Read the model definition and answer for the solid it produces. Units are mm, in the model's axes. A direction names the side the tool comes from. Give positions to 0.01 mm unless a question says otherwise; leave off trailing zeros. Order: outer loops, then holes, each group sorted by start corner. A loop starts at its lowest first (then second) coordinate and runs counter-clockwise, first axis right, second up. Notation, with made-up numbers: M 85,63.25 L 123,63.25 A21 cw 123,93.25 Z; hole C 54,-14.5 d1. An arc over 180 degrees is marked long. One line per item, written item: value.
from build123d import *

# Parameters (mm, degrees)
BOSS_EXTRUDE2_DEPTH = 6


with BuildPart() as part:
    # Sketch1 → Boss-Extrude2 (new body)
    with BuildSketch(Plane(origin=(0, 0, 0), x_dir=(1, 0, 0), z_dir=(0, 1, 0))):
        with BuildLine():
            Line((7.988162854, 331.501326389), (7.988162854, 171.337454215))
            ThreePointArc((7.988162854, 171.337454215), (9.818693497, 167.235107296), (13.984274361, 165.553432905))
            Line((13.984274361, 165.553432905), (49.307855037, 165.553432905))
            Line((49.307855037, 165.553432905), (49.307855037, 163.543518894))
            Line((49.307855037, 163.543518894), (13.984274361, 163.543518894))
            ThreePointArc((13.984274361, 163.543518894), (8.320398521, 165.889579716), (5.974360349, 171.553464938))
            Line((5.974360349, 171.553464938), (5.974999998, 331.501302447))
            ThreePointArc((5.974999998, 331.501302447), (-0.011825567, 337.488163533), (-5.998674291, 331.501325605))
            Line((-5.998674291, 331.501325605), (-5.998674291, 0.561440532))
            ThreePointArc((-5.998674291, 0.561440532), (-0.306028697, -5.993414959), (5.975, 0))
            Line((5.975, 0), (5.975, 115.356719051))
            ThreePointArc((5.975, 115.356719051), (8.250227281, 120.944829403), (13.781744328, 123.354384475))
            Line((13.781744328, 123.354384475), (308.33721248, 123.354384475))
            ThreePointArc((308.33721248, 123.354384475), (313.994066729, 121.011238725), (316.33721248, 115.354384475))
            Line((316.33721248, 115.354384475), (316.33721248, 0.000205216))
            ThreePointArc((316.33721248, 0.000205216), (322.337222061, -5.999794784), (328.33721248, 0.000224379))
            Line((328.33721248, 0.000224379), (328.336683355, 331.50001256))
            ThreePointArc((328.336683355, 331.50001256), (322.26179375, 337.500094056), (316.337490676, 331.351281588))
            Line((316.337490676, 331.351281588), (316.337490676, 171.552255024))
            ThreePointArc((316.337490676, 171.552255024), (313.994332551, 165.895370899), (308.337448427, 163.552212774))
            Line((308.337448427, 163.552212774), (90.793200611, 163.552212774))
            ThreePointArc((90.793200611, 163.552212774), (90.43964722, 163.405766165), (90.293200611, 163.052212774))
            Line((90.293200611, 163.052212774), (90.293200611, 157.424591987))
            Line((90.293200611, 157.424591987), (90.293200611, 154.657877928))
            Line((90.293200611, 154.657877928), (88.293002078, 154.657877928))
            Line((88.293002078, 154.657877928), (88.293002078, 157.424591987))
            Line((88.293002078, 157.424591987), (88.293002078, 163.552212774))
            ThreePointArc((88.293002078, 163.552212774), (88.878788516, 164.966468586), (90.293002078, 165.552255024))
            Line((90.293002078, 165.552255024), (308.337448427, 165.552255024))
            ThreePointArc((308.337448427, 165.552255024), (312.580089114, 167.309614337), (314.337448427, 171.552255024))
            Line((314.337448427, 171.552255024), (314.337448427, 331.693156944))
            ThreePointArc((314.337448427, 331.693156944), (322.432732181, 339.500501309), (330.33721248, 331.500036554))
            Line((330.33721248, 331.500036554), (330.33721248, 0.000205216))
            ThreePointArc((330.33721248, 0.000205216), (322.33721248, -7.999794784), (314.33721248, 0.000205216))
            Line((314.33721248, 0.000205216), (314.33721248, 115.354384475))
            ThreePointArc((314.33721248, 115.354384475), (312.579853167, 119.597025163), (308.33721248, 121.354384475))
            Line((308.33721248, 121.354384475), (13.975047586, 121.356719051))
            ThreePointArc((13.975047586, 121.356719051), (9.732376137, 119.599376562), (7.975, 115.356719051))
            Line((7.975, 115.356719051), (7.975, 0))
            ThreePointArc((7.975, 0), (-0.025317655, -7.999999994), (-8.024999975, 0.000635309))
            Line((-8.024999975, 0.000635309), (-8.011837146, 331.501326389))
            ThreePointArc((-8.011837146, 331.501326389), (-0.011837146, 339.501326389), (7.988162854, 331.501326389))
        make_face()
    extrude(amount=BOSS_EXTRUDE2_DEPTH)


solid = part.part
1) Each of these flat-tipped pins is pushed along its axis until it touches: pin 1 Ø1.8 at (y, z) = (4, -158.5) entering from -X; pin 2 Ø6 at (x, z) = (179, -119.5) entering from -Y; pin 3 Ø3 at (x, y) = (150.5, 1.5) entering from +Z; pin 4 Ø1.8 at (x, y) = (215.5, 3) entering from -Z. Where does it stop, or does it pass through?
Reported:
pin 1: stops at x = -8.02
pin 2: stops at y = 0
pin 3: stops at z = -121.36
pin 4: stops at z = -165.55
2) Which of the six approach directions +Z, -Z, +X, -X, +Y, -Y give full straight-line access (tool end or side, diameter ignored) to faces 4 (the face through (0, 3, 8)), 5 (the face through (8.38, 2.96, -165.83))?
Reported:
face 4: +Z, +Y, -Y
face 5: +Y, -Y
3) Find section D-D, the plane z = -97. Write down the section's boundary in (x, y) (3 decimals), plus the area to 3 significant figures.
Reported:
outline: M -8.021,0 L -5.999,0 L -5.999,6 L -8.021,6 Z; M 5.975,0 L 7.975,0 L 7.975,6 L 5.975,6 Z; M 314.337,0 L 316.337,0 L 316.337,6 L 314.337,6 Z; M 328.337,0 L 330.337,0 L 330.337,6 L 328.337,6 Z
area: 48.1 mm^2
4) Consider probe 1 along X at (y, z) = (5.6, -200.5); probe 2 along Z at (x, y) = (262.5, 3.45); probe 3 along Z at (x, y) = (28, 5.05). Determine where each line is inside the solid, lowest interval first.
Reported:
probe 1: x = -8.02 to -6, 5.97 to 7.99, 314.34 to 316.34, 328.34 to 330.34
probe 2: z = -165.55 to -163.55, -123.35 to -121.35
probe 3: z = -165.55 to -163.54, -123.35 to -121.36
5) Find section A-A, the plane x = 211. Write down the section's boundary in (y, z).
Reported:
outline: M 0,-165.55 L 6,-165.55 L 6,-163.55 L 0,-163.55 Z; M 0,-123.35 L 6,-123.35 L 6,-121.36 L 0,-121.36 Z
6) Determine the mould class of faces 1 (the face through (322.3, 3, -339.5)), 2 (the face through (322.5, 3, 8)), 3 (the face through (314.06, 2.96, -165.96)) for opening direction Z: +Z half, -Z half, draft (parallel to the pull), parting line (faces both ways), or undercut.
Reported:
face 1: -Z half
face 2: +Z half
face 3: undercut
7) Find section B-B, the plane z = -197.5. Write down the section's boundary in (x, y).
Reported:
outline: M -8.02,0 L -6,0 L -6,6 L -8.02,6 Z; M 5.97,0 L 7.99,0 L 7.99,6 L 5.97,6 Z; M 314.34,0 L 316.34,0 L 316.34,6 L 314.34,6 Z; M 328.34,0 L 330.34,0 L 330.34,6 L 328.34,6 Z
